Input: part model. Units: mm. Frame: model coordinates. Face numbers are marked on the shaded views. A direction names the side the tool comes from. Coordinates: 2 decimals unless noted, no trailing zeros. Order: outer loops, then holes, each group sorted by start corner. A loop starts at its lowest first (then second) coordinate and runs counter-clockwise, first axis right, second up. Notation, with made-up numbers: (6.25, 5.5) -> (25.25, 5.5) arc R34 cw to (25.25, 37.5) -> close; hole circle Ø5 at (56, 49.5). An arc over 180 degrees is marked (long way). Use one line per item in the form item = value. Start each with the question number.
1) Pin query (flat end, axial travel): pin 1 (4 mm diameter, centred on y = 3, z = 14, fed in from -X); pin 2 (4 mm diameter, centred on y = -1, z = 15, fed in from +X); pin 3 (2 mm diameter, centred on x = -16.5, z = 10, fed in from +Y). Return the tip coordinate at first contact, or that it passes through.
2) Section query A-A on x = -19.5. Output: boundary loops of the cut face in (y, z).
3) Section query C-C on z = 14.5. Output: boundary loops of the cut face in (x, y), then the cut area to 3 significant figures.
4) Access query for the marked faces 1 and 2. Directions: +Z, -Z, +X, -X, +Y, -Y. A direction counts if a zero-diameter tool reaches every point of the face in a straight line with its end or side. Return the directions, or none.
5) Section query D-D on z = 15.5. Output: boundary loops of the cut face in (x, y).
6) Section query B-B on y = -1. Output: boundary loops of the cut face in (x, z).
7) Ray query, line 1 along Y through (x, z) = (-16.25, 13.25); line 2 along X through (y, z) = (6.5, 14.25); line 3 along Z through (x, y) = (-19, 1.25). Return the intervals inside material, ascending.
from build123d import *

# Parameters (mm, degrees)
SKETCH1_R           = 2
BOSS_EXTRUDE1_DEPTH = 10
BOSS_EXTRUDE4_DEPTH = 4


with BuildPart() as part:
    # Sketch1 → Boss-Extrude1 (new body)
    with BuildSketch(Plane(origin=(0, 0, 0), x_dir=(1, 0, 0), z_dir=(0, 1, 0))):
        with Locations((-18.876405997, -12.710678642)):
            Circle(SKETCH1_R)
    extrude(amount=BOSS_EXTRUDE1_DEPTH)

    # Sketch4 → Boss-Extrude4 (add)
    with BuildSketch(Plane.XZ):
        Polygon((-16.490145939, 16.665308368), (-21.108085773, 16.754555336), (-23.494345831, 12.79992561), (-21.262666056, 8.756048917), (-16.644726221, 8.666801949), (-14.258466163, 12.621431674), align=None)
    extrude(amount=BOSS_EXTRUDE4_DEPTH)


solid = part.part
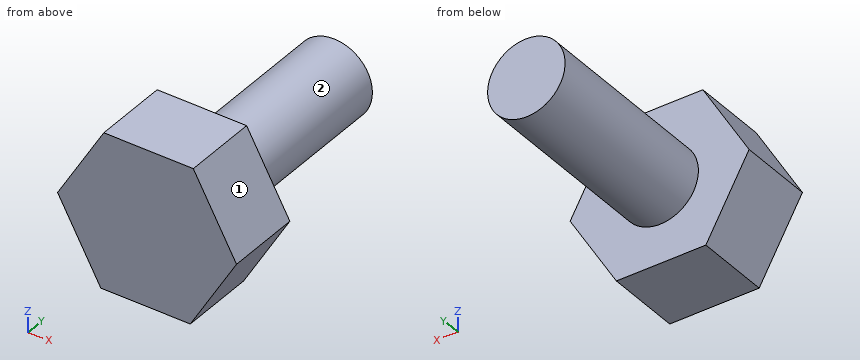
Answers below:
q1.pin_1 = -20.88
q1.pin_2 = -14.47
q1.pin_3 = 0
q2.outline = (-4, 8.72) -> (0, 8.72) -> (0, 10.81) -> (10, 10.81) -> (10, 14.61) -> (0, 14.61) -> (0, 16.72) -> (-4, 16.72) -> close
q3.outline = (-22.47, -4) -> (-15.3, -4) -> (-15.3, 0) -> (-17.98, 0) -> (-17.98, 10) -> (-19.77, 10) -> (-19.77, 0) -> (-22.47, 0) -> close
q3.area = 46.6 mm^2
q4.face_1 = +Z, +X, +Y, -Y
q4.face_2 = +Y
q5.outline = (-21.87, -4) -> (-15.85, -4) -> (-15.85, 0) -> (-21.87, 0) -> close
q6.outline = (-23.49, 12.8) -> (-21.26, 8.76) -> (-16.64, 8.67) -> (-14.26, 12.62) -> (-16.49, 16.67) -> (-21.11, 16.75) -> close
q7.line_1 = -4 to 0
q7.line_2 = -20.15 to -17.6
q7.line_3 = 10.71 to 14.71
